Part model, mm, in its own coordinate system. Face numbers are marked on the shaded views. A direction names the side the tool comes from. Coordinates: 2 decimals unless noted, no trailing zeros. Write each loop counter-clockwise with the first axis right and the second up, starting at its lowest first coordinate (ties: lowest second). Pieces come first, ordered by that corner, then holes. Notation, with made-up numbers: M -16,1.25 L 9,1.25 A14 cw 9,20.25 Z; hole C 55.25,-7 d7. An arc over 180 degrees is marked long. Use a Markdown table: item, result. Add a question column.
Q1. Slice it at C-C on x = -1162.5. Write the cut outline in (y, z), then the cut area to 3 significant figures.
Q2. Pin check, flat tips, straight feed: pin 1 Ø16 at (x, z) = (13.5, -619.5) entering from -Y; pin 2 Ø10 at (x, y) = (-557.5, 404) entering from -Z. Stop position of each tip, or through.
Q3. Wall check: L1, parallel to X at y = 572, z = -372.5; L2, parallel to Z at x = -176, y = 575; L3, parallel to X at y = 1417.5, z = 28. Give the ranges that are in metal, low to high. Write a range as from..to.
Q4. Slice it at D-D on x = -486. Write the cut outline in (y, z), then the cut area to 3 significant figures.
Q5. Slice it at A-A on z = -49. Write the cut outline in (x, y).
Q6. Tool access for the marked faces 4 and 5: list every direction of +Z, -Z, +X, -X, +Y, -Y with a clear straight run to the whole face (end or side of a thin tool).
Q7. Mould opens along X. For the marked faces 1, 2 and 3 say: released by +X, released by -X, zero draft, split by the parting line, or undercut.
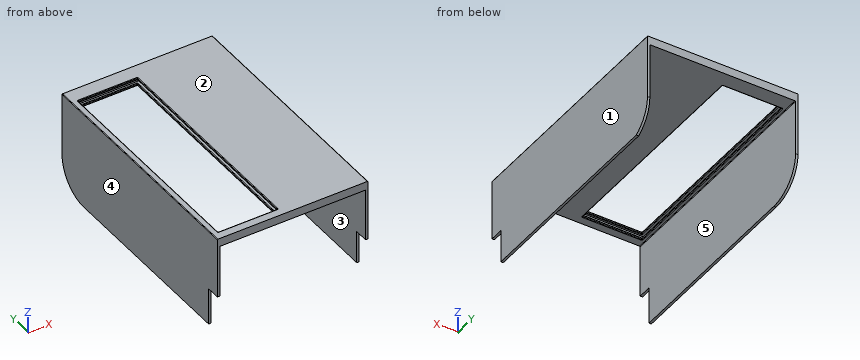
from build123d import *

# Parameters (mm, degrees)
SURFACE_EXTRUDE1_1_DEPTH = 2027
THICKEN1_T2              = 20
CUT_EXTRUDE1_REACH       = 2504.773
SKETCH3_W                = 500
SKETCH3_H                = 1900
CUT_EXTRUDE2_DEPTH       = 20
BOSS_EXTRUDE1_DEPTH      = 50
SKETCH7_W                = 70
SKETCH7_H                = 70
BOSS_EXTRUDE2_DEPTH      = 500
CUT_EXTRUDE3_DEPTH       = 523
CUT_EXTRUDE3_DEPTH_BACK  = 645
SKETCH6_W                = 30
SKETCH6_H                = 1870
FILLET1_R                = 5
CUT_EXTRUDE4_REACH       = 2504.773
SKETCH9_W                = 20
SKETCH9_H                = 36
CUT_EXTRUDE5_DEPTH       = 1996


with BuildPart() as body_1:
    # Surface-Extrude1: a surface, the sketch's curves swept straight by 2027 mm
    with BuildLine(Plane(origin=(0, 0, 0), x_dir=(1, 0, 0), z_dir=(0, 1, 0)), mode=Mode.PRIVATE) as surface_extrude1_1_path:
        Line((-1222, 750), (-1222, 0))
        Line((-1222, 0), (0, 0))
        Line((0, 0), (0, 750))
    surface_extrude1_1 = Shell.extrude(surface_extrude1_1_path.wire(), (0 * SURFACE_EXTRUDE1_1_DEPTH, 1 * SURFACE_EXTRUDE1_1_DEPTH, 0 * SURFACE_EXTRUDE1_1_DEPTH))
    add(Solid.thicken(surface_extrude1_1, -THICKEN1_T2))

    # Cut-Extrude1: up to this face of the body (flat: up to its plane)
    cut_extrude1_end = Plane(body_1.part.faces().sort_by_distance((-1242, 1013.5, -365))[0])
    # Sketch2 → Cut-Extrude1 (cut, up to the picked face)
    with BuildSketch(Plane(origin=(20, 0, 0), x_dir=(0, 0, -1), z_dir=(1, 0, 0)), mode=Mode.PRIVATE) as cut_extrude1_sk1:
        with BuildLine():
            Line((466, 2027), (750, 2027))
            Line((750, 2027), (750, 1743))
            ThreePointArc((750, 1743), (666.818325857, 1943.818325857), (466, 2027))
        make_face()
    cut_extrude1_tool1 = split(extrude(cut_extrude1_sk1.sketch, amount=-CUT_EXTRUDE1_REACH, mode=Mode.PRIVATE), bisect_by=cut_extrude1_end, keep=Keep.BOTH, mode=Mode.PRIVATE)
    add(cut_extrude1_tool1.solids().sort_by(Axis((20, 1963.563505, -686.563505), (-1, 0, 0)))[0], mode=Mode.SUBTRACT)

    # Sketch3 → Cut-Extrude2 (cut)
    with BuildSketch(Plane.XY.offset(20)):
        with Locations((-942, 950)):
            Rectangle(SKETCH3_W, SKETCH3_H)
    extrude(amount=-CUT_EXTRUDE2_DEPTH, mode=Mode.SUBTRACT)

    # Sketch5 → Boss-Extrude1 (add)
    with BuildSketch(Plane.XY.offset(20)):
        Polygon((20, 0), (20, 2027), (-1242, 2027), (-1242, 0), (-1192, 0), (-1192, 1900), (-692, 1900), (-692, 0), align=None)
    extrude(amount=BOSS_EXTRUDE1_DEPTH)

    # Sketch7 → Boss-Extrude2 (add)
    with BuildSketch(Plane(origin=(-1192, 0, 0), x_dir=(0, 0, -1), z_dir=(1, 0, 0))):
        with Locations((-35, 35)):
            Rectangle(SKETCH7_W, SKETCH7_H)
    extrude(amount=BOSS_EXTRUDE2_DEPTH)

    # Sketch6 → Cut-Extrude3 (cut, two sides: drawn at the far end of the back side and taken through both)
    with BuildSketch(Plane.ZY.offset(692).offset(-CUT_EXTRUDE3_DEPTH_BACK)):
        with Locations((35, 985)):
            Rectangle(SKETCH6_W, SKETCH6_H)
    extrude(amount=CUT_EXTRUDE3_DEPTH + CUT_EXTRUDE3_DEPTH_BACK, mode=Mode.SUBTRACT)

    # Fillet1
    fillet1_edges = [body_1.edges().sort_by_distance(p)[0] for p in [
        (-1242, 1013.5, 70),
        (-942, 1900, 70),
        (-692, 985, 70),
        (-1192, 985, 70),
        (-692, 985, 0),
        (-942, 70, 70),
        (-942, 70, 0),
        (-1192, 70, 10),
        (-692, 70, 10),
        (-692, 70, 60),
        (-1192, 70, 60),
        (-942, 70, 50),
        (-942, 70, 20),
        (-692, 1900, 60),
        (-1192, 1900, 60),
        (-1192, 985, 20),
        (-942, 1900, 20),
        (-692, 985, 20),
        (-692, 985, 50),
        (-942, 1900, 50),
        (-1192, 985, 50),
        (0, 1013.5, 0),
        (-1222, 1013.5, 0),
        (-692, 1900, 10),
        (-942, 1900, 0),
        (-1192, 1900, 10),
        (-1192, 985, 0),
        (20, 1013.5, 70),
    ]]
    fillet(fillet1_edges, radius=FILLET1_R)

    # Sketch8 → Cut-Extrude4 (cut, up to next)
    with BuildSketch(Plane(origin=(20, 0, 0), x_dir=(0, 0, -1), z_dir=(1, 0, 0)), mode=Mode.PRIVATE) as cut_extrude4_sk1:
        Polygon((439, 0), (439.023010168, 115), (750, 115), (750, 0), align=None)
    cut_extrude4_tool1 = extrude(cut_extrude4_sk1.sketch, amount=-CUT_EXTRUDE4_REACH, mode=Mode.PRIVATE) & body_1.part
    add(cut_extrude4_tool1.solids().sort_by_distance((20, 57.499291, -594.505752))[0], mode=Mode.SUBTRACT)
    add(cut_extrude4_tool1.solids().sort_by_distance((20, 57.499291, -594.505752))[1], mode=Mode.SUBTRACT)

    # Sketch9 → Cut-Extrude5 (cut)
    with BuildSketch(Plane(origin=(0, 0, 0), x_dir=(1, 0, 0), z_dir=(0, 1, 0))):
        with Locations((10, 732)):
            Rectangle(SKETCH9_W, SKETCH9_H)
    extrude(amount=CUT_EXTRUDE5_DEPTH, mode=Mode.SUBTRACT)


solid = body_1.part
Recorded:
| question | item | result |
|---|---|---|
| 1 | outline | M 0,0 L 65,0 A5 ccw 70,5 L 70,15 A5 ccw 65,20 L 50,20 L 50,50 L 65,50 A5 ccw 70,55 L 70,65 A5 ccw 65,70 L 0,70 Z; M 1900,5 A5 ccw 1905,0 L 2027,0 L 2027,70 L 1905,70 A5 ccw 1900,65 L 1900,55 A5 ccw 1905,50 L 1920,50 L 1920,20 L 1905,20 A5 ccw 1900,15 Z |
| 1 | area | 12,500 mm² |
| 2 | pin 1 | y = 115 |
| 2 | pin 2 | z = 0 |
| 3 | L1 | -1242..-1222, 0..20 |
| 3 | L2 | 0..20, 50..70 |
| 3 | L3 | -1242..-1215, -47..20 |
| 4 | outline | M 0,0 L 2027,0 L 2027,70 L 0,70 Z; hole M 50,20 L 1920,20 L 1920,50 L 50,50 Z |
| 4 | area | 85,800 mm² |
| 5 | outline | M -1242,0 L -1222,0 L -1222,2027 L -1242,2027 Z; M 0,0 L 20,0 L 20,2027 L 0,2027 Z |
| 6 | face 4 | +Z, -Z, -X, +Y, -Y |
| 6 | face 5 | -Z, +Y, -Y |
| 7 | face 1 | released by +X |
| 7 | face 2 | zero draft |
| 7 | face 3 | undercut |
